Here's how the part is built. I have some questions about the finished solid (model axes, mm). A direction names the side the tool comes from. Give positions to 0.01 mm unless a question says otherwise; leave off trailing zeros. Loops run counter-clockwise (first coordinate to the right, second up) from the corner with the lowest first, then second, coordinate; pieces in that order, holes last.
Q1. Will these pins go through, and if not, where does the flat tip stop? P1, Ø1, axis at x = -2.5, y = -2.5, coming from the -Z side; P2, Ø2.5, axis at x = 0, y = 0, coming from the +Z side; P3, Ø1, axis at y = -1, z = 32, coming from the +X side.
Q2. We'd pull the mould along X, two halves only. Please class faces 3 (the face through (-2.986, 1.756, 36.989)), 4 (the face through (2.986, -1.756, 36.989)), 5 (the face through (1, -2, 67)): +X half, -X half, draft (parallel to the pull), parting line (faces both ways), or undercut.
Q3. If we section it at B-B (z = 41): Please give me the cut outline in (x, y).
Q4. If we section it at A-A (z = 67): Please give me the cut outline in (x, y), plus the area to 3 significant figures.
Q5. I need wall thicknesses on line 1 (X direction, y = 2.65, z = 67); line 2 (Y direction, x = 1, z = 69); line 3 (Z direction, x = 0, y = 2.2). Which ranges of each line are inside material? Lowest first, please.
Q6. For faces 1 (the face through (-3.014, -1.708, 36.989)), 2 (the face through (1.6, 0.07, 66.89)), which set-ups out of +Z, -Z, +X, -X, +Y, -Y let a thin tool reach every point of the face, with its end or its side?
from build123d import *

# Parameters (mm, degrees)
F1_DEPTH = 75
F3_D     = 3.2
F3_DEPTH = 16
F3_TIP   = 0.9613769904
F5_D     = 2
F5_DEPTH = 20
F5_TIP   = 0.600860619
F6_SIZE  = 1


with BuildPart() as f1:
    # F0 (on Top) → F1 (new body)
    with BuildSketch(Plane.XY):
        Polygon((-2, -3.4641016151), (2, -3.4641016151), (4, 0), (2, 3.4641016151), (-2, 3.4641016151), (-4, 0), align=None)
    extrude(amount=F1_DEPTH)

    # F3
    with Locations(Plane.XY.offset(75)):
        with Locations((0, 0)):
            Hole(F3_D / 2, depth=F3_DEPTH)
            with Locations((0, 0, -(F3_DEPTH + F3_TIP / 2))):  # 118° drill point
                Cone(0, F3_D / 2, F3_TIP, mode=Mode.SUBTRACT)

    # F5
    with Locations(Plane(origin=(0, 3.4641016151, 0), x_dir=(-1, 0, 0), z_dir=(0, 1, 0))):
        with Locations((0, 67)):
            Hole(F5_D / 2, depth=F5_DEPTH)
            with Locations((0, 0, -(F5_DEPTH + F5_TIP / 2))):  # 118° drill point
                Cone(0, F5_D / 2, F5_TIP, mode=Mode.SUBTRACT)

    # F6
    f6_edges = [f1.edges().sort_by_distance(p)[0] for p in [
        (0, 3.464102, 75),
        (-3, 1.732051, 75),
        (-3, -1.732051, 75),
        (0, -3.464102, 75),
        (3, -1.732051, 75),
        (3, 1.732051, 75),
        (-3, 1.732051, 0),
        (0, 3.464102, 0),
        (-3, -1.732051, 0),
        (0, -3.464102, 0),
        (3, -1.732051, 0),
        (3, 1.732051, 0),
    ]]
    chamfer(f6_edges, length=F6_SIZE)


solid = f1.part
Check sheet entries:
1. P1: stops at z = 0.45
1. P2: stops at z = 58.79
1. P3: stops at x = 3.71
2. face 3: -X half
2. face 4: +X half
2. face 5: undercut
3. outline: (-4, 0) - (-2, -3.46) - (2, -3.46) - (4, 0) - (2, 3.46) - (-2, 3.46) - close
4. outline: (-4, 0) - (-2, -3.46) - (-1, -3.46) - (-1, -1.25) arc R1.6 cw to (-1, 1.25) - (-1, 3.46) - (-2, 3.46) - close; (1, -3.46) - (2, -3.46) - (4, 0) - (2, 3.46) - (1, 3.46) - (1, 1.25) arc R1.6 cw to (1, -1.25) - close
4. area: 25.6 mm2
5. line 1: x = -2.47 to -1, 1 to 2.47
5. line 2: y = -3.46 to -1.25, 1.25 to 3.46
5. line 3: z = 0 to 66, 68 to 75
6. face 1: +Z, -Z, -X, -Y
6. face 2: +Z
